Autodesk Fusion 360 part; units mm, degrees
sketch "Sketch1" plane through (0, 0, 0) normal (0, 1, 0) x (1, 0, 0)
  line L0 (0, 0) -> (35, 0)
  line L1 (35, 0) -> (35, -35)
  line L2 (35, -35) -> (0, -35)
  line L3 (0, -35) -> (0, 0)
  line L4 (3.2, -3.2) -> (31.8, -3.2)
  line L5 (31.8, -3.2) -> (31.8, -31.8)
  line L6 (31.8, -31.8) -> (3.2, -31.8)
  line L7 (3.2, -31.8) -> (3.2, -3.2)
  dimension "d1" = 35
  dimension "d2" = 3.2
  dimension "d3" = 3.2
  dimension "d4" = 35
  dimension "d5" = 3.2
  dimension "d6" = 3.2
extrude "Extrude1" add sketch "Sketch1" along normal blind 35 makes body 1
sketch "Sketch2" plane through (0, 35, 0) normal (0, 1, 0) x (-1, 0, 0)
  line L0 (-31.8, 31.8) -> (-3.2, 31.8)
  line L1 (-3.2, 31.8) -> (-3.2, 3.2)
  line L2 (-3.2, 3.2) -> (-31.8, 3.2)
  line L3 (-31.8, 3.2) -> (-31.8, 31.8)
  line L4 (0, 35) -> (-35, 35)
  line L5 (-35, 35) -> (-35, 0)
  line L6 (-35, 0) -> (0, 0)
  line L7 (0, 0) -> (0, 35)
  line L8 (2.5, -2.5) -> (-37.5, -2.5)
  line L9 (-37.5, -2.5) -> (-37.5, 37.5)
  line L10 (-37.5, 37.5) -> (2.5, 37.5)
  line L11 (2.5, 37.5) -> (2.5, -2.5)
  line L12 (-26.8, 30.8) -> (-19.3, 30.8)
  line L13 (-19.3, 30.8) -> (-19.3, 23.3)
  line L14 (-19.3, 23.3) -> (-26.8, 23.3)
  line L15 (-26.8, 23.3) -> (-26.8, 30.8)
  line L16 (-31.8, 31.8) -> (-3.2, 31.8)
  line L17 (-31.8, 3.2) -> (-31.8, 31.8)
  dimension "d9" = 2.5
  dimension "d10" = 2.5
  dimension "d11" = 2.5
  dimension "d12" = 2.5
  dimension "d54" = 7.5
  dimension "d55" = 7.5
  dimension "d56" = 1
  dimension "d57" = 5
sketch "Sketch3" plane through (0, 35, 0) normal (0, 1, 0) x (-1, 0, 0)
sketch "Sketch4" plane through (0, 0, 0) normal (-1, 0, 0) x (0, 0, 1)
  line L0 (0, 0) -> (35, 0)
  line L1 (35, 0) -> (35, 35)
  line L2 (35, 35) -> (0, 35)
  line L3 (0, 35) -> (0, 0)
  line L4 (-2.5, 35) -> (7.5, 35)
  arc A0 (-2.5, 35) -> (7.5, 35) centre (2.5, 35.0004) ccw
  arc A1 (7.5, 35) -> (17.5, 35) centre (12.5, 35) ccw
  arc A2 (17.5, 35) -> (27.5, 35) centre (22.5, 35) ccw
  line L5 (27.5, 35) -> (27.5, 35)
  line L6 (-2.5, 35) -> (5, 45)
  line L7 (5, 45) -> (30, 45)
  line L8 (5, 23.2) -> (15, 23.2)
  line L9 (15, 23.2) -> (15, 3.2)
  line L10 (15, 3.2) -> (5, 3.2)
  line L11 (5, 3.2) -> (5, 23.2)
  line L12 (20, 23.2) -> (30, 23.2)
  line L13 (30, 23.2) -> (30, 13.2)
  line L14 (30, 13.2) -> (20, 13.2)
  line L15 (20, 13.2) -> (20, 23.2)
  line L16 (7.5, 35) -> (17.5, 35)
  line L17 (27.5, 35) -> (17.5, 35)
  line L18 (35, 35) -> (37.5, 35)
  arc A3 (27.5, 35) -> (37.5, 35) centre (32.5, 35) ccw
  line L19 (37.5, 35) -> (30, 45)
  line L20 (37.5, 35) -> (-2.5, 35)
  point P0 (35, 35)
  point P1 (37.5, 35)
  dimension "d13" = 10
  dimension "d14" = 5
  dimension "d15" = 10
  dimension "d16" = 10
  dimension "d18" = 7.5
  dimension "d22" = 10
  dimension "d23" = 20
  dimension "d24" = 3.2
  dimension "d25" = 5
  dimension "d26" = 5
  dimension "d27" = 10
  dimension "d28" = 10
  dimension "d29" = 13.2
  dimension "d31" = 10
  dimension "d33" = 7.5
  dimension "d35" = 40
  dimension "d36" = 10
extrude "Extrude2" add sketch "Sketch1" along normal blind 3.2 contours L4 L5 L6 L7 bodies 1
extrude "Extrude3" cut sketch "Sketch4" against normal blind 3.2 contours L8 L9 L10 L11 bodies 1
extrude "Extrude4" cut sketch "Sketch4" against normal blind 3.2 contours L12 L13 L14 L15 bodies 1
extrude "Extrude5" add sketch "Sketch4" along normal blind 2.5 separate body contours L3 L4 A0 L20 | L2 L3 L4 A0 L20 | L1 L2 A3 L20 | L1 L18 A3 L20 | L2 L4 L6 L7 L16 L17 L18 L19 L20 | L2 A1 L16 L20 | L2 A2 L17 L20 makes body 2
extrude "Extrude6" add sketch "Sketch4" against normal blind 37.5 contours L3 L4 A0 L20 bodies 1 2
extrude "Extrude7" add sketch "Sketch4" against normal blind 37.5 separate body contours L1 L18 A3 L20 makes body 3
extrude "Extrude8" add sketch "Sketch4" against normal blind 37.5 contours L2 L4 L6 L7 L16 L17 L18 L19 L20 bodies 1 3
extrude "Extrude9" add sketch "Sketch4" against normal blind 2.5 from surface at -35 contours L2 L3 L4 A0 L20 | L1 L2 A3 L20 | L2 A1 L16 L20 | L2 A2 L17 L20 bodies 1
extrude "Extrude10" add sketch "Sketch2" along normal blind 18 contours L12 L13 L14 L15 bodies 1
Here's how the part is built. I have some questions about the finished solid (model axes, mm). A direction names the side the tool comes from. Give positions to 0.01 mm unless a question says otherwise; leave off trailing zeros. Loops run counter-clockwise (first coordinate to the right, second up) from the corner with the lowest first, then second, coordinate; pieces in that order, holes last. Notation, with made-up numbers: (24, 37.5) -> (34, 37.5) arc R31 ccw to (34, 64.5) -> close; hole circle Ø2 at (-0.5, 74). An arc over 180 degrees is marked (long way). Use one line per item in the form item = value. Start each with the question number.
1) For P1, Ø1.6, axis at x = 1.5, y = 16, coming from the +Z side; P2, Ø1, axis at x = 2, y = 11, coming from the -Z side; P3, Ø1.5, axis at y = 30, z = 6.5, coming from the -X side, each with a flat end and sliding along its axis, tell me the tip position at first contact or that it passes through.
2) Imagine slicing it at B-B (x = 1). Please give me the cut outline in (y, z).
3) Thinking about a two-plate mould opening in Y: for faces 4 (the face through (26.8, 49, 27)), 5 (the face through (2, 13, 15)), 6 (the face through (23, 53, 27)), 7 (the face through (18, 35, 18)), which applies, +Y half, -Y half, draft (parallel to the pull), parting line (faces both ways), or undercut?
4) Which directions (+Z, -Z, +X, -X, +Y, -Y) give clear straight access to the entire face, cutting with the end or side of a thin tool? Please do faces 1 (the face through (17, 15, 0)), 2 (the face through (23, 48, 30.8)), 3 (the face through (2, 23.2, 10)).
5) Please list where these lines run through material, in increasing order: line 1 along Y through (x, z) = (8, 6.5); line 2 along X through (y, z) = (29, 14).
6) Imagine slicing it at D-D (z = 22.5). Please give me the cut outline in (x, y), then the cut area to 3 significant figures.
7) Imagine slicing it at A-A (x = 12). Please give me the cut outline in (y, z), then the cut area to 3 significant figures.
Check values:
q1.P1 = 35
q1.P2 = 0
q1.P3 = 0
q2.outline = (0, 0) -> (30.67, 0) arc R5 ccw to (35, -2.5) -> (45, 5) -> (45, 30) -> (35, 37.5) arc R5 ccw to (30.67, 35) -> (0, 35) -> close; hole (3.2, 5) -> (23.2, 5) -> (23.2, 15) -> (3.2, 15) -> close; hole (13.2, 20) -> (23.2, 20) -> (23.2, 30) -> (13.2, 30) -> close
q3.face_4 = draft
q3.face_5 = undercut
q3.face_6 = +Y half
q3.face_7 = undercut
q4.face_1 = -Z, +X, -X, -Y
q4.face_2 = +Z, +X, -X, +Y
q4.face_3 = -X
q5.line_1 = 0 to 3.2, 35 to 45
q5.line_2 = 0 to 3.2, 31.8 to 35
q6.outline = (-2.5, 30) -> (0, 30) -> (0, 23.2) -> (3.2, 23.2) -> (3.2, 35) -> (31.8, 35) -> (31.8, 3.2) -> (3.2, 3.2) -> (3.2, 13.2) -> (0, 13.2) -> (0, 0) -> (35, 0) -> (35, 30) -> (37.5, 30) -> (37.5, 45) -> (-2.5, 45) -> close
q6.area = 709 mm^2
q7.outline = (0, 0) -> (30.67, 0) arc R5 ccw to (35, -2.5) -> (45, 5) -> (45, 30) -> (35, 37.5) arc R5 ccw to (30.67, 35) -> (0, 35) -> close; hole (3.2, 3.2) -> (35, 3.2) -> (35, 31.8) -> (3.2, 31.8) -> close
q7.area = 656 mm^2
